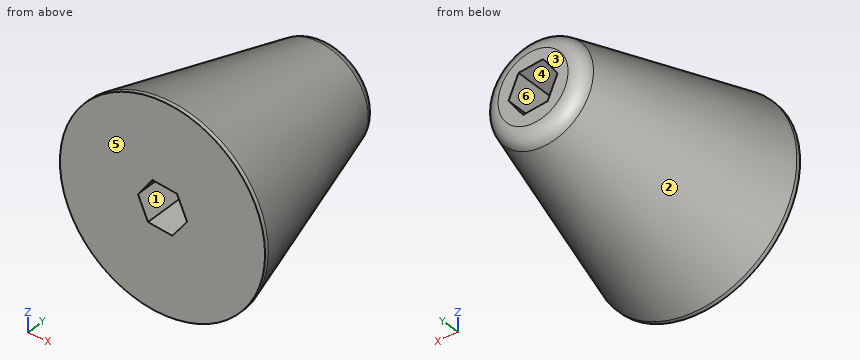
from build123d import *

# Parameters (mm, degrees)
SKETCH2_R               = 31.75
BOSS_EXTRUDE1_DEPTH     = 63.5
BOSS_EXTRUDE1_TAPER     = 15
SKETCH3_R               = 31.75
BOSS_EXTRUDE2_DEPTH     = 1.27
CUT_EXTRUDE2_DEPTH      = 64.5000001
CUT_EXTRUDE2_DEPTH_BACK = 2.27
FILLET1_R               = 5.08


with BuildPart() as part:
    # Sketch2 → Boss-Extrude1 (new body)
    with BuildSketch(Plane(origin=(0, 0, 0), x_dir=(1, 0, 0), z_dir=(0, 1, 0))):
        Circle(SKETCH2_R)
    extrude(amount=BOSS_EXTRUDE1_DEPTH, taper=BOSS_EXTRUDE1_TAPER)

    # Sketch3 → Boss-Extrude2 (add)
    with BuildSketch(Plane.XZ):
        Circle(SKETCH3_R)
    extrude(amount=BOSS_EXTRUDE2_DEPTH)

    # Sketch7 → Cut-Extrude2 (cut, two sides)
    with BuildSketch(Plane(origin=(0, 0, 0), x_dir=(1, 0, 0), z_dir=(0, 1, 0))) as cut_extrude2_sk:
        Polygon((4.482800658, -6.168866962), (7.583795831, 0.79778577), (3.100995172, 6.966652731), (-4.482800658, 6.168866962), (-7.583795831, -0.79778577), (-3.100995172, -6.966652731), align=None)
    extrude(amount=CUT_EXTRUDE2_DEPTH, mode=Mode.SUBTRACT)
    extrude(cut_extrude2_sk.sketch, amount=-CUT_EXTRUDE2_DEPTH_BACK, mode=Mode.SUBTRACT)

    # Fillet1
    fillet1_edges = [part.edges().sort_by_distance(p)[0] for p in [
        (-14.735226281, 63.5, 0),
    ]]
    fillet(fillet1_edges, radius=FILLET1_R)


solid = part.part
Verification items for the finished model (mm, model axes). Face numbers are marked on the shaded views. A direction names the side the tool comes from. Coordinates: 2 decimals unless noted, no trailing zeros. Order: outer loops, then holes, each group sorted by start corner. A loop starts at its lowest first (then second) coordinate and runs counter-clockwise, first axis right, second up. Notation, with made-up numbers: M -23.75,78.25 L 25.25,78.25 A31 ccw 25.25,112.25 Z; hole C 68,60 d9. An arc over 180 degrees is marked long. One line per item, written item: value. Start each with the question number.
Item 1: Sectioned sample at A-A (x = 0). Enter the section's corners in (y, z), then the cut area to 3 significant figures.
Item 2: Access from +Z, -Z, +X, -X, +Y, -Y to the whole of each face (thin tool, end or side, straight path). Record for the marked faces 5 and 6.
Item 3: Scan lines: probe 1 along Z at (x, y) = (-5, 27); probe 2 along Z at (x, y) = (4.5, 48.5); probe 3 along X at (y, z) = (49.5, -5). Record each from-to range of solid material in increasing order.
Item 4: Mould release check, pull along X, two halves, no side actions. Record for the marked faces 1, 2, 3 and 4: released by +X, released by -X, zero draft, split by the parting line, or undercut.
Item 5: Gauge pin test, flat ends, axial feed: pin 1 (1 mm diameter, centred on x = -21.5, y = 28.5, fed in from -Z); pin 2 (10 mm diameter, centred on x = 4.5, y = 19.5, fed in from +Z); pin 3 (4 mm diameter, centred on x = -9.5, y = 33, fed in from +Z); pin 4 (1 mm diameter, centred on y = 46, z = -22, fed in from +X). Record the tip position at first contact, or that the pin passes through.
Item 6: Sectioned sample at B-B (y = 44). Enter the section's corners in (x, z).
Item 7: Sectioned sample at C-C (y = 26). Enter the section's corners in (x, z).
Conclusion:
1. outline: M -1.27,-31.75 L 0,-31.75 L 59.73,-15.74 A5.08 ccw 63.5,-10.84 L 63.5,-6.64 L -1.27,-6.64 Z; M -1.27,6.64 L 63.5,6.64 L 63.5,10.84 A5.08 ccw 59.73,15.74 L 0,31.75 L -1.27,31.75 Z
1. area: 2,170 mm^2
2. face 5: +Z, -Z, +X, -X, -Y
2. face 6: +Y, -Y
3. probe 1: z = -24 to -5.01, 4.35 to 24
3. probe 2: z = -18.21 to -5.04, 6.13 to 18.21
3. probe 3: x = -17.8 to -5, 4.53 to 17.8
4. face 1: undercut
4. face 2: split by the parting line
4. face 3: zero draft
4. face 4: undercut
5. pin 1: stops at z = -11.89
5. pin 2: stops at z = 27.64
5. pin 3: stops at z = 21.84
5. pin 4: passes through
6. outline: C 0,0 d39.92; hole M -7.58,0.8 L -4.48,-6.17 L 3.1,-6.97 L 7.58,-0.8 L 4.48,6.17 L -3.1,6.97 Z
7. outline: C 0,0 d49.57; hole M -7.58,0.8 L -4.48,-6.17 L 3.1,-6.97 L 7.58,-0.8 L 4.48,6.17 L -3.1,6.97 Z
